Could you check a few things on this model? Use its own coordinates, in mm. A direction names the side the tool comes from. Give positions to 0.01 mm unless a question says otherwise; leave off trailing zeros. Order: outer loops, then holes, each group sorted by start corner. A loop starts at its lowest first (then second) coordinate and runs counter-clockwise, first axis right, second up. Notation, with made-up numbers: M -27,-3.75 L -7,-3.75 A23 cw -7,20.25 Z; hole C -35,12.25 d7. An arc over 180 degrees is marked long. Use a Markdown table: item, result. Add a question column.
Item 1: If we mould it in two halves opening along Z, with no side actions, what happens to faces 5 (the face through (15.47, 1.48, -1.15)), 6 (the face through (-29.83, 0.6, 0.23)), 7 (the face through (0.4, 0.6, 17.63))? For each: released by +Z, released by -Z, zero draft, split by the parting line, or undercut.
Item 2: For faces 1 (the face through (15, 3, -1)), 2 (the face through (8.38, 5.74, 0.19)), 3 (the face through (-15, 8, 1)), 4 (the face through (15, 29.4, 16)), which set-ups out of +Z, -Z, +X, -X, +Y, -Y let a thin tool reach every point of the face, with its end or its side?
Item 3: Suppose I cut it at C-C on z = 0. Count the separate pieces of the cut face and the enclosed holes in it, plus the area to 3 significant figures.
Item 4: Suppose I cut it at D-D on z = 14. Write out the boundary of the cut face in (x, y), plus the area to 3 significant figures.
Item 5: Suppose I cut it at B-B on y = 11. Write out the boundary of the cut face in (x, z).
Item 6: If I drill on L1, parallel to X at y = 6, z = 0 (3 decimals); L2, parallel to Z at x = -12.7, y = 6.1 (3 decimals); L3, parallel to Z at x = -12.7, y = 6.7 (3 decimals), over which ranges is the centre line in solid material (lowest first)? Write a range as from..to.
Item 7: Suppose I cut it at A-A on x = 12.7. Write out the boundary of the cut face in (y, z) (3 decimals), plus the area to 3 significant figures.
Item 8: I'm going to push flat-ended pins straight in: pin 1 Ø2.5 at (y, z) = (19, -15) entering from +X; pin 2 Ø6 at (y, z) = (14, -8.5) entering from +X; pin 3 Ø1 at (x, z) = (-16.5, -6) entering from +Y; pin 4 Ø1.5 at (y, z) = (12.5, 16.5) entering from -X. Where does each tip first touch, or does it pass through?
Autodesk Inventor part; units mm, degrees
ref_plane "YZ Plane" through (0, 0, 0) normal (1, 0, 0) x (0, 1, 0)
ref_plane "XZ Plane" through (0, 0, 0) normal (0, 1, 0) x (-1, 0, 0)
ref_plane "XY Plane" through (0, 0, 0) normal (0, 0, 1) x (1, 0, 0)
sketch "Sketch1" plane through (0, 0, 0) normal (0, 1, 0) x (-1, 0, 0)
  line L0 (30.4, 18.2) -> (-30.4, 18.2)
  line L1 (-30.4, 18.2) -> (-30.4, -18.2)
  line L2 (-30.4, -18.2) -> (30.4, -18.2)
  line L3 (30.4, -18.2) -> (30.4, 18.2)
  point P0 (0, 0)
  dimension "d0" = 60.8
  dimension "d1" = 36.4
extrude "Extrusion1" add sketch "Sketch1" along normal blind 5
sketch "Sketch2" plane through (0, 5, 0) normal (0, 1, 0) x (1, 0, 0)
  line L0 (30.4, 18.2) -> (-30.4, 18.2)
  line L1 (-30.4, 18.2) -> (-0.4, 18.2)
  line L2 (-0.4, 18.2) -> (-0.4, 13.2)
  line L3 (-0.4, 13.2) -> (-30.4, 13.2)
  line L4 (-30.4, 13.2) -> (-30.4, 18.2)
  line L5 (30.4, -18.2) -> (30.4, 18.2)
  line L6 (30.4, -18.2) -> (0.4, -18.2)
  line L7 (0.4, -18.2) -> (0.4, -13.2)
  line L8 (0.4, -13.2) -> (30.4, -13.2)
  line L9 (30.4, -13.2) -> (30.4, -18.2)
  point P0 (0, 0)
  dimension "d4" = 30
  dimension "d5" = 5
  dimension "d6" = 30
  dimension "d7" = 5
extrude "Extrusion2" add sketch "Sketch2" along normal blind 24.4
sketch "Sketch3" plane through (0, 5, 0) normal (0, 1, 0) x (1, 0, 0)
  circle A0 centre (12.7, 0) radius 4.325
  circle A1 centre (-12.7, 0) radius 4.325
  point P0 (0, 0)
  dimension "d10" = 8.65
  dimension "d11" = 8.65
extrude "Extrusion3" add sketch "Sketch3" along normal blind 3
sketch "Sketch4" plane through (-12.7, 8, 0) normal (0, 1, 0) x (1, 0, 0)
  circle A0 centre (0, 0) radius 2
  circle A1 centre (25.4, 0) radius 4.325
  circle A2 centre (25.4, 0) radius 2
  point P0 (12.7, 0)
  dimension "d14" = 4
  dimension "d15" = 4
extrude "Extrusion4" cut sketch "Sketch4" against normal blind 15 contours A0 | A2
sketch "Sketch5" plane through (0, 0, 0) normal (0, -1, 0) x (1, 0, 0)
  circle A0 centre (12.7, 0) radius 2
  circle A1 centre (12.7, 0) radius 3
  circle A2 centre (-12.7, 0) radius 2
  circle A3 centre (-12.7, 0) radius 3
  point P0 (0, 0)
  dimension "d18" = 6
  dimension "d19" = 6
extrude "Extrusion5" cut sketch "Sketch5" against normal blind 3 contours A0 | A1 | A2 | A3
chamfer "Chamfer1" distance 1.5 angle 45 2 edges at (8.375, 8, 0) (-17.025, 8, 0)
fillet "Fillet1" radius 2 8 edges at (0, 0, 18.2) (-30.4, 0, 0) (0, 0, -18.2) (30.4, 0, 0) (-30.4, 14.7, -18.2) (-30.4, 2.5, 18.2) (30.4, 14.7, 18.2) (30.4, 2.5, -18.2)
properties part number "2Wide5mm"
Findings below:
| question | item | result |
|---|---|---|
| 1 | face 5 | undercut |
| 1 | face 6 | zero draft |
| 1 | face 7 | released by +Z |
| 2 | face 1 | -Y |
| 2 | face 2 | +Y |
| 2 | face 3 | +Z, +X, -X, +Y |
| 2 | face 4 | +Z, -Z, +X, -X, +Y |
| 3 | separate pieces | 3 |
| 3 | enclosed holes | 0 |
| 3 | area | 274 mm^2 |
| 4 | outline | M -30.4,2 A2 ccw -28.4,0 L 28.4,0 A2 ccw 30.4,2 L 30.4,29.4 L 0.4,29.4 L 0.4,5 L -30.4,5 Z |
| 4 | area | 1,030 mm^2 |
| 5 | outline | M -30.4,-16.2 A2 ccw -28.4,-18.2 L -0.4,-18.2 L -0.4,-13.2 L -30.4,-13.2 Z; M 0.4,13.2 L 30.4,13.2 L 30.4,16.2 A2 ccw 28.4,18.2 L 0.4,18.2 Z |
| 6 | L1 | x = -17.025..-14.7, -10.7..-8.375, 8.375..10.7, 14.7..17.025 |
| 6 | L2 | z = -18.2..-13.2, -4.325..-2, 2..4.325 |
| 6 | L3 | z = -18.2..-13.2, -4.125..-2, 2..4.125 |
| 7 | outline | M 0,-16.2 A2 ccw 2,-18.2 L 5,-18.2 L 5,-4.325 L 6.5,-4.325 L 8,-2.825 L 8,-2 L 3,-2 L 3,-3 L 0,-3 Z; M 0,3 L 3,3 L 3,2 L 8,2 L 8,2.825 L 6.5,4.325 L 5,4.325 L 5,13.2 L 29.4,13.2 L 29.4,18.2 L 2,18.2 A2 ccw 0,16.2 Z |
| 7 | area | 288 mm^2 |
| 8 | pin 1 | stops at x = -0.4 |
| 8 | pin 2 | passes through |
| 8 | pin 3 | stops at y = 5 |
| 8 | pin 4 | stops at x = 0.4 |
